Build history of the part. All positions in model axes, mm. A direction names the side the tool comes from. Give positions to 0.01 mm unless a question says otherwise; leave off trailing zeros. Write each loop counter-clockwise with the first axis right and the second up, starting at its lowest first coordinate (ties: lowest second). Pieces come first, ordered by that corner, then holes. Notation, with made-up numbers: (52.25, 71.25) - (99.25, 71.25) arc R13 ccw to (99.25, 94.25) - close; hole circle Ø1 at (10.5, 52). An arc over 180 degrees is marked (long way). Use one line per item in the form item = value. Start each with the question number.
from build123d import *

# Parameters (mm, degrees)
BASE_DEPTH            = 1
SKETCH2_R             = 5
BLISTER_EXTRUDE_DEPTH = 3
BLISTER_PATTERN_COUNT = 4
BLISTER_PATTERN_PITCH = 12.3


with BuildPart() as part:
    # Sketch1 → Base (new body)
    with BuildSketch(Plane(origin=(0, 0, 0), x_dir=(1, 0, 0), z_dir=(0, 1, 0))):
        with BuildLine():
            Line((-44, -33.5), (44, -33.5))
            ThreePointArc((44, -33.5), (47.535533906, -32.035533906), (49, -28.5))
            Line((49, -28.5), (49, 28.5))
            ThreePointArc((49, 28.5), (47.535533906, 32.035533906), (44, 33.5))
            Line((44, 33.5), (-44, 33.5))
            ThreePointArc((-44, 33.5), (-47.535533906, 32.035533906), (-49, 28.5))
            Line((-49, 28.5), (-49, -28.5))
            ThreePointArc((-49, -28.5), (-47.535533906, -32.035533906), (-44, -33.5))
        make_face()
    extrude(amount=BASE_DEPTH)

    # Sketch2 → Blister-Extrude (add)
    with BuildSketch(Plane(origin=(0, 1, 0), x_dir=(1, 0, 0), z_dir=(0, 1, 0))):
        with Locations(Location((-37, -23.5, 0), (0, 0, 270))):
            Circle(SKETCH2_R)
        with Locations(Location((-24.75, -23.5, 0), (0, 0, 270))):
            Circle(SKETCH2_R)
        with Locations(Location((-12.5, -23.5, 0), (0, 0, 270))):
            Circle(SKETCH2_R)
        with Locations(Location((-0.25, -23.5, 0), (0, 0, 270))):
            Circle(SKETCH2_R)
        with Locations(Location((12, -23.5, 0), (0, 0, 270))):
            Circle(SKETCH2_R)
        with Locations(Location((24.25, -23.5, 0), (0, 0, 270))):
            Circle(SKETCH2_R)
        with Locations(Location((36.5, -23.5, 0), (0, 0, 270))):
            Circle(SKETCH2_R)
    blister_extrude = extrude(amount=BLISTER_EXTRUDE_DEPTH)

    # Blister-Pattern: Blister-Extrude ×4
    with Locations(*[(0, 0, -i * BLISTER_PATTERN_PITCH) for i in range(1, BLISTER_PATTERN_COUNT)]):
        add(blister_extrude)


solid = part.part
(1) Cut at A-A, the plane y = 2.3. State how many separate pieces and enclosed holes the cut face has, then the cut area to 3 significant figures.
(2) Pin check, flat tips, straight feed: pin 1 Ø2 at (x, z) = (24.5, -21.5) entering from -Y; pin 2 Ø1.5 at (x, y) = (-35.5, 2) entering from -Z. Stop position of each tip, or through.
(3) Cut at D-D, the plane z = -25. Give the cut face in (x, y), then the cut area to 3 significant figures.
(4) Which spindle directions (+Z, -Z, +X, -X, +Y, -Y) get a long thin tool onto all of the face, cutting with end or side? Do faces 4 (the cylindrical face through (19.37, 2.48, -2.18)), 5 (the flat face through (-37, 4, 11)). Say none if no direction does.
(5) Two-plate mould, pull along Z, no slides. Class faces 1 (the cylindrical face through (47.57, 0.49, -32)), 2 (the flat face through (12, 4, -13)), 3 (the cylindrical face through (-36.78, 2.479, 6.205)): +Z half, -Z half, draft (parallel to the pull), parting line (faces both ways), or undercut.
(6) Wall check: line 1 (Z direction, x = 25.5, y = 1.35); line 2 (Z direction, x = -15, y = 3.85); line 3 (Y direction, x = -34.5, z = 4). Give the ranges that are in metal, low to high. Write a range as from..to.
(7) Cut at C-C, the plane x = 24.25. Give the cut face in (y, z), then the cut area to 3 significant figures.
Solution:
q1.separate_pieces = 28
q1.enclosed_holes = 0
q1.area = 2,200 mm2
q2.pin_1 = 0
q2.pin_2 = -18.34
q3.outline = (-49, 0) - (49, 0) - (49, 1) - (-49, 1) - close
q3.area = 98.0 mm2
q4.face_4 = +Y
q4.face_5 = +Z, -Z, +X, -X, +Y
q5.face_1 = -Z half
q5.face_2 = draft
q5.face_3 = undercut
q6.line_1 = -18.24..-8.56, -5.94..3.74, 6.36..16.04, 18.66..28.34
q6.line_2 = -17.73..-9.07, -5.43..3.23, 6.87..15.53, 19.17..27.83
q6.line_3 = 0..1
q7.outline = (0, -33.5) - (1, -33.5) - (1, -18.4) - (4, -18.4) - (4, -8.4) - (1, -8.4) - (1, -6.1) - (4, -6.1) - (4, 3.9) - (1, 3.9) - (1, 6.2) - (4, 6.2) - (4, 16.2) - (1, 16.2) - (1, 18.5) - (4, 18.5) - (4, 28.5) - (1, 28.5) - (1, 33.5) - (0, 33.5) - close
q7.area = 187 mm2
